from build123d import *

# Parameters (mm, degrees)
F1_DEPTH = 50
F2_R     = 16.25
F3_DEPTH = 50.001
F4_R     = 1.7
F5_DEPTH = 15.561876
F6_R     = 3


with BuildPart() as f1:
    # F0 (on Front) → F1 (new body)
    with BuildSketch(Plane.XZ):
        with BuildLine():
            Line((-21.273122, 9.52742), (28.726878, 9.52742))
            Line((28.726878, 9.52742), (28.726878, 24.52742))
            ThreePointArc((28.726878, 24.52742), (3.729103, 25.077618), (-21.273122, 24.794238))
            Line((-21.273122, 24.794238), (-21.273122, 9.52742))
        make_face()
    extrude(amount=F1_DEPTH)

    # F2 (on face) → F3 (cut, through all)
    with BuildSketch(Plane.YZ.offset(28.726878)):
        with Locations((-25, 3.52742)):
            Circle(F2_R)
    extrude(amount=-F3_DEPTH, mode=Mode.SUBTRACT)

    # F4 (on face) → F5 (cut, through all)
    with BuildSketch(Plane(origin=(0, 0, 9.52742), x_dir=(1, 0, 0), z_dir=(0, 0, -1))):
        with Locations((-16.273122, 45)):
            Circle(F4_R)
        with Locations((23.726878, 45)):
            Circle(F4_R)
        with Locations((-16.273122, 5)):
            Circle(F4_R)
        with Locations((23.726878, 5)):
            Circle(F4_R)
    extrude(amount=-F5_DEPTH, mode=Mode.SUBTRACT)

    # F6
    f6_edges = [f1.edges().sort_by_distance(p)[0] for p in [
        (28.726878, -50, 17.02742),
        (-21.273122, -50, 17.160829),
        (-21.273122, 0, 17.160829),
        (28.726878, 0, 17.02742),
    ]]
    fillet(f6_edges, radius=F6_R)


solid = f1.part
Input: part model. Units: mm. Frame: model coordinates. A direction names the side the tool comes from. Give positions to 0.01 mm unless a question says otherwise; leave off trailing zeros. Loops run counter-clockwise (first coordinate to the right, second up) from the corner with the lowest first, then second, coordinate; pieces in that order, holes last. Notation, with made-up numbers: (89.5, -30.75) -> (133.5, -30.75) arc R26 cw to (133.5, 3.25) -> close; hole circle Ø5 at (61.25, 66). An arc over 180 degrees is marked (long way). Answer as a JSON object with one key per item and string values. Group by question number.
Item 1: Line query: probe 1 along X at (y, z) = (-45, 20); probe 2 along X at (y, z) = (-6.5, 23.5); probe 3 along Z at (x, y) = (2, -44.5). Output: solid intervals per line, ascending.
Item 2: Cut plane A-A, the plane z = 23.25. Return the cut outline in (x, y).
Item 3: Reachability of faces 1 (the cylindrical face through (-20.418, -49.098, 17.092)), 2 (the cylindrical face through (4.079, -24.65, 25.076)) from +Z, -Z, +X, -X, +Y, -Y: full face, straight path, thin tool, end or side. Return the list, or none.
Item 4: Cut plane B-B, the plane z = 18.25. Return the cut outline in (x, y).
Item 5: Pin query (flat end, axial travel): P1, Ø1.5, axis at x = -9.5, y = -40.5, coming from the +Z side; P2, Ø4, axis at x = 23.73, y = -5, coming from the +Z side. Return the tip coordinate at first contact, or that it passes through.
Item 6: Pull-direction query (Y, two-part tool) for faces 3 (the flat face through (3, -50, 17)), 4 (the cylindrical face through (-17.622, -43.966, 17.132)), 5 (the flat face through (3, -5, 9.527)); classes: released by +Y, released by -Y, zero draft, split by the parting line, or undercut.
Item 7: Cut plane D-D, the plane z = 13.75. Return the cut outline in (x, y).
Item 8: Cut plane C-C, the plane y = -44. Return the cut outline in (x, z).
Checks:
{
 "1": {"probe 1": "x = -21.27 to -17.97, -14.57 to 22.03, 25.43 to 28.73", "probe 2": "x = -21.27 to -17.07, -15.47 to 22.93, 24.53 to 28.73", "probe 3": "z = 9.53 to 25.08"},
 "2": {"outline": "(-21.27, -47) arc R3 ccw to (-18.27, -50) -> (25.73, -50) arc R3 ccw to (28.73, -47) -> (28.73, -3) arc R3 ccw to (25.73, 0) -> (-18.27, 0) arc R3 ccw to (-21.27, -3) -> close; hole circle Ø3.4 at (-16.27, -45); hole circle Ø3.4 at (-16.27, -5); hole circle Ø3.4 at (23.73, -45); hole circle Ø3.4 at (23.73, -5)"},
 "3": {"face 1": "+Z, -Z, -X, -Y", "face 2": "+Z, +Y, -Y"},
 "4": {"outline": "(-21.27, -47) arc R3 ccw to (-18.27, -50) -> (25.73, -50) arc R3 ccw to (28.73, -47) -> (28.73, -31.88) -> (-21.27, -31.88) -> close; (-21.27, -18.12) -> (28.73, -18.12) -> (28.73, -3) arc R3 ccw to (25.73, 0) -> (-18.27, 0) arc R3 ccw to (-21.27, -3) -> close; hole circle Ø3.4 at (-16.27, -45); hole circle Ø3.4 at (-16.27, -5); hole circle Ø3.4 at (23.73, -45); hole circle Ø3.4 at (23.73, -5)"},
 "5": {"P1": "stops at z = 25.04", "P2": "stops at z = 24.77"},
 "6": {"face 3": "released by -Y", "face 4": "undercut", "face 5": "zero draft"},
 "7": {"outline": "(-21.27, -47) arc R3 ccw to (-18.27, -50) -> (25.73, -50) arc R3 ccw to (28.73, -47) -> (28.73, -37.63) -> (-21.27, -37.63) -> close; (-21.27, -12.37) -> (28.73, -12.37) -> (28.73, -3) arc R3 ccw to (25.73, 0) -> (-18.27, 0) arc R3 ccw to (-21.27, -3) -> close; hole circle Ø3.4 at (-16.27, -45); hole circle Ø3.4 at (-16.27, -5); hole circle Ø3.4 at (23.73, -45); hole circle Ø3.4 at (23.73, -5)"},
 "8": {"outline": "(-21.27, 9.53) -> (-17.65, 9.53) -> (-17.65, 24.89) arc R750 ccw to (-21.27, 24.79) -> close; (-14.9, 9.53) -> (22.35, 9.53) -> (22.35, 24.75) arc R750 ccw to (-14.9, 24.95) -> close; (25.1, 9.53) -> (28.73, 9.53) -> (28.73, 24.53) arc R750 ccw to (25.1, 24.66) -> close"}
}
